The model under review builds one solid part; all positions refer to its coordinate system, in mm. Give positions to 0.01 mm unless a question says otherwise; leave off trailing zeros. Order: outer loops, then holes, each group sorted by start corner. A loop starts at its lowest first (then second) coordinate and runs counter-clockwise, first axis right, second up.
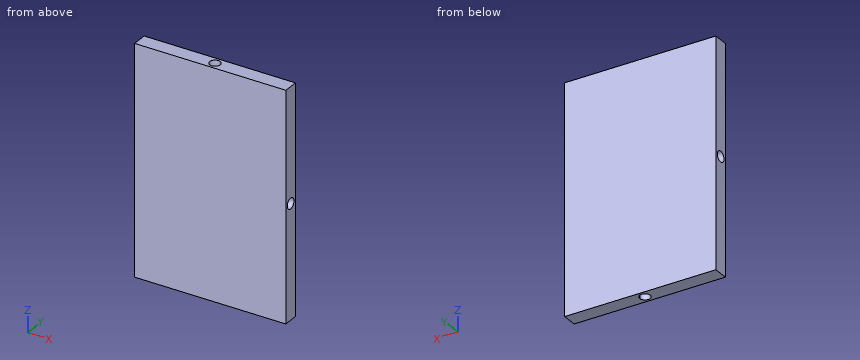
```python
from build123d import *

# Parameters (mm, degrees)
SKETCH_1_W          = 100
SKETCH_1_H          = 150
EXTRUDE_1_DEPTH     = 10
SKETCH_2_R          = 3.5
CUT_EXTRUDE_1_DEPTH = 10
SKETCH_3_R          = 3.5
CUT_EXTRUDE_2_DEPTH = 10
CUT_EXTRUDE_3_DEPTH = 10
SKETCH_5_R          = 3.5
CUT_EXTRUDE_4_DEPTH = 10


with BuildPart() as part:
    # 草图1 → 凸台-拉伸1 (new body)
    with BuildSketch(Plane(origin=(0, 0, 0), x_dir=(1, 0, 0), z_dir=(0, 1, 0))):
        Rectangle(SKETCH_1_W, SKETCH_1_H)
    extrude(amount=EXTRUDE_1_DEPTH)

    # 草图2 → 切除-拉伸1 (cut)
    with BuildSketch(Plane.XY.offset(75)):
        with Locations((0, 5)):
            Circle(SKETCH_2_R)
    extrude(amount=-CUT_EXTRUDE_1_DEPTH, mode=Mode.SUBTRACT)

    # 草图3 → 切除-拉伸2 (cut)
    with BuildSketch(Plane(origin=(50, 0, 0), x_dir=(0, 0, -1), z_dir=(1, 0, 0))):
        with Locations((0, 5)):
            Circle(SKETCH_3_R)
    extrude(amount=-CUT_EXTRUDE_2_DEPTH, mode=Mode.SUBTRACT)

    # 草图4 → 切除-拉伸3 (cut)
    with BuildSketch(Plane(origin=(0, 0, -75), x_dir=(-1, 0, 0), z_dir=(0, 0, -1))):
        with BuildLine():
            ThreePointArc((3.482630166, 5.348263017), (0, 8.5), (-3.482630166, 5.348263017))
            Line((-3.482630166, 5.348263017), (0, 5))
            Line((0, 5), (3.482630166, 5.348263017))
        make_face()
        with BuildLine():
            Line((0, 5), (-3.482630166, 5.348263017))
            ThreePointArc((-3.482630166, 5.348263017), (-3.5, 5), (-3.482630166, 4.651736983))
            Line((-3.482630166, 4.651736983), (0, 5))
        make_face()
        with BuildLine():
            Line((3.482630166, 5.348263017), (0, 5))
            Line((0, 5), (3.482630166, 4.651736983))
            ThreePointArc((3.482630166, 4.651736983), (3.495654844, 4.825652043), (3.5, 5))
            ThreePointArc((3.5, 5), (3.495654844, 5.174347957), (3.482630166, 5.348263017))
        make_face()
        with BuildLine():
            Line((3.482630166, 4.651736983), (0, 5))
            Line((0, 5), (-3.482630166, 4.651736983))
            ThreePointArc((-3.482630166, 4.651736983), (0, 1.5), (3.482630166, 4.651736983))
        make_face()
    extrude(amount=-CUT_EXTRUDE_3_DEPTH, mode=Mode.SUBTRACT)

    # 草图5 → 切除-拉伸4 (cut)
    with BuildSketch(Plane.ZY.offset(50)):
        with Locations((0, 5)):
            Circle(SKETCH_5_R)
    extrude(amount=-CUT_EXTRUDE_4_DEPTH, mode=Mode.SUBTRACT)


solid = part.part
```
Item 1: Clearance check with a flat-ended pin moving along its axis: pin 1 Ø5.5 at (y, z) = (5, 0) entering from +X. State where the tip first meets the part, or that it passes through.
Values found:
pin 1: stops at x = 40
Item 2: Take a section at A-A (x = 0). Give the boundary of the cut face in (y, z).
Values found:
outline: (0, -75) - (1.5, -75) - (1.5, -65) - (8.5, -65) - (8.5, -75) - (10, -75) - (10, 75) - (8.5, 75) - (8.5, 65) - (1.5, 65) - (1.5, 75) - (0, 75) - close
Item 3: Take a section at C-C (x = -44). Give the boundary of the cut face in (y, z).
Values found:
outline: (0, -75) - (10, -75) - (10, 75) - (0, 75) - close; hole circle Ø7 at (5, 0)
Item 4: For line 1 (Y direction, x = -45, z = 0); line 2 (X direction, y = 4, z = 1.5), list the stretches that pass through material, from the lowest coordinate up.
Values found:
line 1: y = 0 to 1.5, 8.5 to 10
line 2: x = -40 to 40
Item 5: Take a section at D-D (y = 3). Give the boundary of the cut face in (x, z).
Values found:
outline: (-50, -75) - (-2.87, -75) - (-2.87, -65) - (2.87, -65) - (2.87, -75) - (50, -75) - (50, -2.87) - (40, -2.87) - (40, 2.87) - (50, 2.87) - (50, 75) - (2.87, 75) - (2.87, 65) - (-2.87, 65) - (-2.87, 75) - (-50, 75) - (-50, 2.87) - (-40, 2.87) - (-40, -2.87) - (-50, -2.87) - close
Item 6: Take a section at B-B (z = 0). Give the boundary of the cut face in (x, y).
Values found:
outline: (-50, 0) - (50, 0) - (50, 1.5) - (40, 1.5) - (40, 8.5) - (50, 8.5) - (50, 10) - (-50, 10) - (-50, 8.5) - (-40, 8.5) - (-40, 1.5) - (-50, 1.5) - close
